```python
from build123d import *

# Parameters (mm, degrees)
SKETCH1_R           = 61.5
BOSS_EXTRUDE1_DEPTH = 5
BOSS_EXTRUDE1_DRAFT = -5
SKETCH2_R           = 2.5
SKETCH2_R_2         = 5
CUT_EXTRUDE2_DEPTH  = 88.117736426
SKETCH3_R           = 20
CUT_EXTRUDE3_DEPTH  = 2


with BuildPart() as part:
    # Sketch1 → Boss-Extrude1 (with draft: the straight prism first)
    with BuildSketch(Plane(origin=(0, 0, 0), x_dir=(1, 0, 0), z_dir=(0, 1, 0))):
        Circle(SKETCH1_R)
    extrude(amount=-BOSS_EXTRUDE1_DEPTH)
    # Boss-Extrude1: the draft: its side faces are tilted about the plane it starts from
    boss_extrude1_sides = [part.faces().sort_by_distance(p)[0] for p in [
        (-61.5, -2.5, 0),
    ]]
    draft(boss_extrude1_sides, Plane(origin=(0, 0, 0), x_dir=(1, 0, 0), z_dir=(0, 1, 0)), BOSS_EXTRUDE1_DRAFT)

    # Sketch2 → Cut-Extrude2 (cut, through all)
    with BuildSketch(Plane(origin=(0, 0, 0), x_dir=(1, 0, 0), z_dir=(0, 1, 0))):
        with Locations(Location((23.62, 23.62, 0), (0, 0, 270))):
            Circle(SKETCH2_R)
        with Locations(Location((23.62, -23.62, 0), (0, 0, 270))):
            Circle(SKETCH2_R)
        with Locations(Location((-23.62, -23.62, 0), (0, 0, 270))):
            Circle(SKETCH2_R)
        with Locations(Location((-23.62, 23.62, 0), (0, 0, 270))):
            Circle(SKETCH2_R)
        with Locations(Location((0, 0, 0), (0, 0, 270))):
            Circle(SKETCH2_R_2)
    extrude(amount=-CUT_EXTRUDE2_DEPTH, mode=Mode.SUBTRACT)

    # Sketch3 → Cut-Extrude3 (cut)
    with BuildSketch(Plane(origin=(0, 0, 0), x_dir=(1, 0, 0), z_dir=(0, 1, 0))):
        with Locations(Location((0, 0, 0), (0, 0, 270))):
            Circle(SKETCH3_R)
    extrude(amount=-CUT_EXTRUDE3_DEPTH, mode=Mode.SUBTRACT)


solid = part.part
```
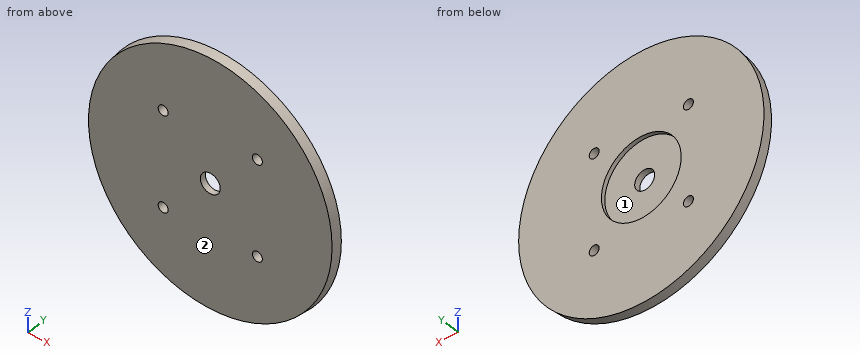
Geometry check sheet. Reference: the model listing, model coordinates, mm. Face numbers are marked on the shaded views. Give positions to 0.01 mm unless a question says otherwise; leave off trailing zeros. Order: outer loops, then holes, each group sorted by start corner. A loop starts at its lowest first (then second) coordinate and runs counter-clockwise, first axis right, second up. Notation, with made-up numbers: (-12, 10.25) -> (28, 10.25) arc R26 ccw to (28, 49.25) -> close; hole circle Ø1 at (0, 75.5). An arc over 180 degrees is marked (long way). Write each question's results on one line, items separated by ' | '. Start each with the question number.
(1) Gauge pin test, flat end, axial feed: P1, Ø2, axis at y = -2.5, z = -44.5, coming from the +X side. Record the tip position at first contact, or that the pin passes through.
(2) Scan lines: line 1 (X direction, y = -2.2, z = 22); line 2 (X direction, y = -0.25, z = -4); line 3 (X direction, y = -2.2, z = -23.62). Record each from-to range of solid material in increasing order.
(3) Sectioned sample at B-B (y = -3.9). Enter the section's corners in (x, z).
(4) Sectioned sample at A-A (x = 0). Enter the section's corners in (y, z), plus the area to 3 significant figures.
(5) Mould release check, pull along Z, two halves, no side actions. Record for the marked faces 1 and 2: pulls with the +Z half, pulls with the -Z half, needs draft (parallel to the pull), parting line crosses it, or undercut.
(6) Sectioned sample at C-C (x = -23.62). Give the number of separate pieces and of enclosed holes in the cut face, plus the area to 3 significant figures.
Answer below:
1) P1: x = 43.17
2) line 1: -57.22 to -25.52, -21.72 to 21.72, 25.52 to 57.22 | line 2: -61.35 to -19.6, 19.6 to 61.35 | line 3: -56.57 to -26.12, -21.12 to 21.12, 26.12 to 56.57
3) outline: circle Ø122.32 at (0, 0); hole circle Ø5 at (-23.62, -23.62); hole circle Ø5 at (-23.62, 23.62); hole circle Ø10 at (0, 0); hole circle Ø5 at (23.62, -23.62); hole circle Ø5 at (23.62, 23.62)
4) outline: (-5, -61.06) -> (0, -61.5) -> (0, -20) -> (-2, -20) -> (-2, -5) -> (-5, -5) -> close; (-5, 5) -> (-2, 5) -> (-2, 20) -> (0, 20) -> (0, 61.5) -> (-5, 61.06) -> close | area: 503 mm2
5) face 1: undercut | face 2: needs draft
6) separate pieces: 3 | enclosed holes: 0 | area: 515 mm2
